Drawing for the job (mm, zero at the part's lowest x, y, z). A direction names the side the tool comes from. Give positions to 0.01 mm unless a question says otherwise; leave off trailing zeros. Order: outer loops, then holes, each group sorted by start corner. A loop starts at its lowest first (then second) coordinate and runs counter-clockwise, first axis right, second up. Notation, with made-up numbers: (46.5, 27) -> (57.5, 27) arc R27 cw to (57.5, 46) -> close; hole circle Ø8 at (-38.5, 46). An arc over 180 degrees is marked (long way). Use a Markdown table: item, result. Add a question column.
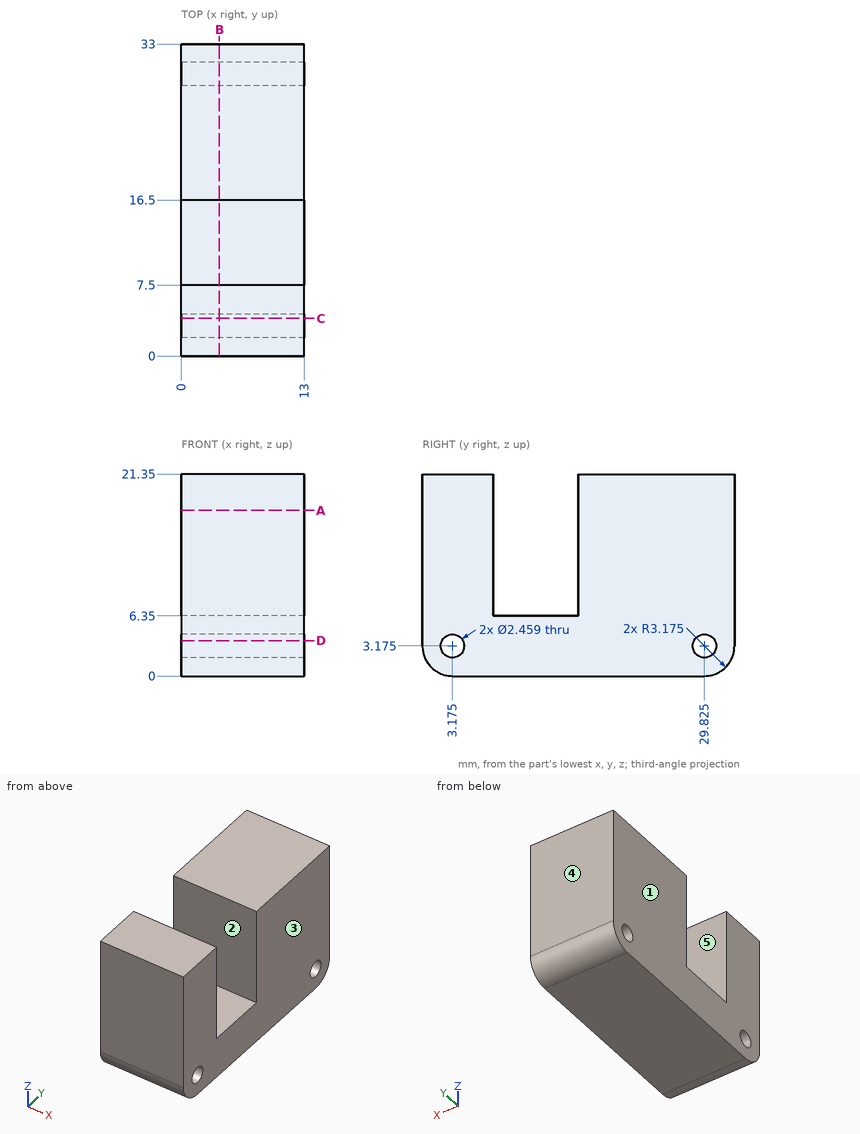
(1) Band-saw the part on C-C on y = 4. Give the cut face in (x, z), plus the area to 3 significant figures.
(2) Band-saw the part on A-A on z = 17.5. Give the cut face in (x, y).
(3) Mould opens along Y. For the marked faces 3, 4 and 5 say: released by +Y, released by -Y, zero draft, split by the parting line, or undercut.
(4) Band-saw the part on D-D on z = 3.75. Give the cut face in (x, y), plus the area to 3 significant figures.
(5) Band-saw the part on B-B on x = 4. State how many separate pieces and enclosed holes the cut face has, plus the area to 3 significant figures.
(6) Tool access for the marked faces 1 and 2: list every direction of +Z, -Z, +X, -X, +Y, -Y with a clear straight run to the whole face (end or side of a thin tool).
(7) Wall check: probe 1 along Y at (x, z) = (1.75, 11); probe 2 along Y at (x, z) = (5.5, 3); probe 3 along Y at (x, z) = (4.5, 2.75). Give the ranges that are in metal, low to high.
Response:
| question | item | result |
|---|---|---|
| 1 | outline | (0, 0) -> (13, 0) -> (13, 2.26) -> (0, 2.26) -> close; (0, 4.09) -> (13, 4.09) -> (13, 21.35) -> (0, 21.35) -> close |
| 1 | area | 254 mm² |
| 2 | outline | (0, 0) -> (13, 0) -> (13, 7.5) -> (0, 7.5) -> close; (0, 16.5) -> (13, 16.5) -> (13, 33) -> (0, 33) -> close |
| 3 | face 3 | zero draft |
| 3 | face 4 | released by +Y |
| 3 | face 5 | undercut |
| 4 | outline | (0, 0) -> (13, 0) -> (13, 2.09) -> (0, 2.09) -> close; (0, 4.26) -> (13, 4.26) -> (13, 28.74) -> (0, 28.74) -> close; (0, 30.91) -> (13, 30.91) -> (13, 33) -> (0, 33) -> close |
| 4 | area | 372 mm² |
| 5 | separate pieces | 1 |
| 5 | enclosed holes | 2 |
| 5 | area | 556 mm² |
| 6 | face 1 | +Z, -Z, -X, +Y, -Y |
| 6 | face 2 | +Z, +X, -X |
| 7 | probe 1 | y = 0 to 7.5, 16.5 to 33 |
| 7 | probe 2 | y = 0 to 1.96, 4.39 to 28.61, 31.04 to 33 |
| 7 | probe 3 | y = 0.03 to 2.02, 4.33 to 28.67, 30.98 to 32.97 |
